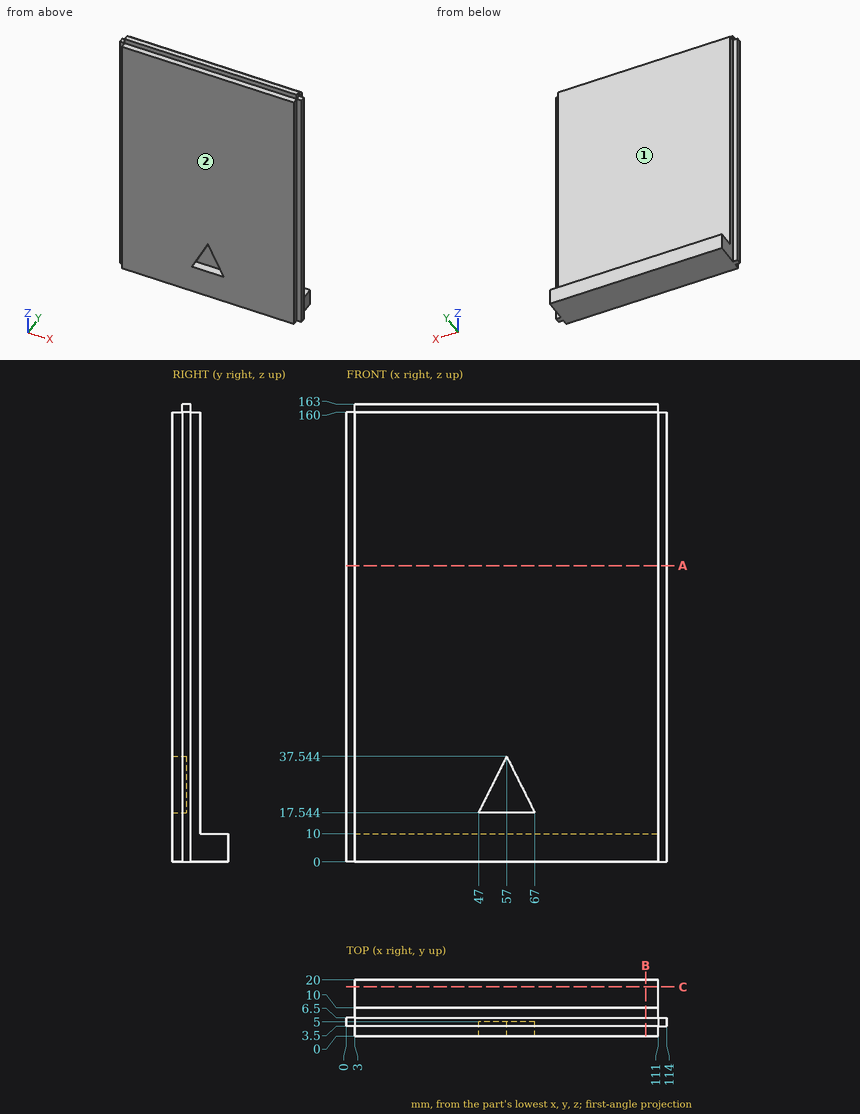
Job drawing, mm, ordinate dimensions from the low corner. One solid piece. A direction names the side the tool comes from. Round coordinates to 2 decimals unless told otherwise and drop trailing zeros. Loops run counter-clockwise (first coordinate to the right, second up) from the corner with the lowest first, then second, coordinate; pieces in that order, holes last. Notation, with made-up numbers: M 15,78.5 L 31,78.5 A27 cw 31,99.5 Z; hole C 35,50.25 d6. An arc over 180 degrees is marked long. One line per question, with ' | ' between items. Start each with the question number.
Item 1: Cut at B-B, the plane x = 106.5. Write the cut outline in (y, z), plus the area to 3 significant figures.
Item 2: Wall check: line 1 (Y direction, x = 93, z = 73); line 2 (X direction, y = 8, z = 91). Give the ranges that are in metal, low to high.
Item 3: Which spindle directions (+Z, -Z, +X, -X, +Y, -Y) get a long thin tool onto all of the face, cutting with end or side? Do the marked faces 1 and 2. Say none if no direction does.
Item 4: Pin check, flat tips, straight feed: pin 1 Ø3.5 at (x, z) = (112.5, 60.5) entering from +Y; pin 2 Ø10 at (x, y) = (23.5, 17.5) entering from -Z; pin 3 Ø1.8 at (y, z) = (2, 100) entering from +X; pin 4 Ø1.5 at (x, z) = (71.5, 161) entering from -Y. Stop position of each tip, or through.
Item 5: Cut at A-A, the plane z = 105.5. Write the cut outline in (x, y), plus the area to 3 significant figures.
Item 6: Cut at C-C, the plane y = 17.5. Write the cut outline in (x, z).
Responses:
1) outline: M 0,0 L 20,0 L 20,10 L 10,10 L 10,160 L 6.5,160 L 6.5,163 L 3.5,163 L 3.5,160 L 0,160 Z | area: 1,710 mm²
2) line 1: y = 0 to 10 | line 2: x = 3 to 111
3) face 1: +Z, +X, -X, +Y | face 2: +Z, -Z, +X, -X, -Y
4) pin 1: stops at y = 10 | pin 2: stops at z = 0 | pin 3: stops at x = 111 | pin 4: stops at y = 3.5
5) outline: M 0,3.5 L 3,3.5 L 3,0 L 111,0 L 111,3.5 L 114,3.5 L 114,6.5 L 111,6.5 L 111,10 L 3,10 L 3,6.5 L 0,6.5 Z | area: 1,100 mm²
6) outline: M 3,0 L 111,0 L 111,10 L 3,10 Z
